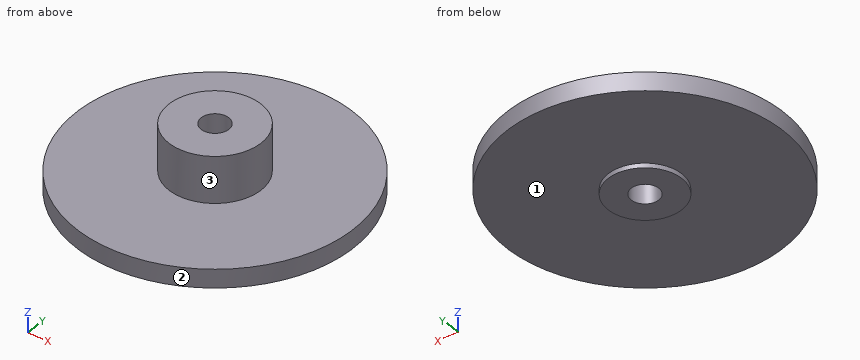
Autodesk Inventor part; units mm, degrees
ref_plane "YZ Plane" through (0, 0, 0) normal (1, 0, 0) x (0, 1, 0)
ref_plane "XZ Plane" through (0, 0, 0) normal (0, 1, 0) x (-1, 0, 0)
ref_plane "XY Plane" through (0, 0, 0) normal (0, 0, 1) x (1, 0, 0)
sketch "スケッチ1" plane through (0, 0, 0) normal (0, 0, 1) x (1, 0, 0)
  circle A0 centre (0, 0) radius 15
  dimension "d0" = 30
extrude "押し出し1" add sketch "スケッチ1" along normal blind 2
sketch "スケッチ2" plane through (0, 0, 2) normal (0, 0, 1) x (1, 0, 0)
  circle A0 centre (0, 0) radius 5
  dimension "d3" = 10
extrude "押し出し2" add sketch "スケッチ2" along normal blind 5
sketch "スケッチ4" plane through (0, 0, 0) normal (0, 0, -1) x (-1, 0, 0)
  circle A0 centre (0, 0) radius 4
  dimension "d9" = 8
extrude "押し出し4" add sketch "スケッチ4" along normal blind 0.5
sketch "スケッチ5" plane through (0, 0, 7) normal (0, 0, 1) x (1, 0, 0)
  circle A0 centre (0, 0) radius 1.5
  dimension "d12" = 3
extrude "押し出し5" cut sketch "スケッチ5" against normal blind 15
properties part number "Gear2_BSS0.5-30A" material "真鍮"
Geometry: final body of the model. Coordinates: model frame, mm. Face numbers are marked on the shaded views. A direction names the side the tool comes from. Give positions to 0.01 mm unless a question says otherwise; leave off trailing zeros. Loops run counter-clockwise (first coordinate to the right, second up) from the corner with the lowest first, then second, coordinate; pieces in that order, holes last. Notation, with made-up numbers: (50.5, 28.25) - (86.5, 28.25) arc R34 cw to (86.5, 63.25) - close; hole circle Ø1 at (-29, 85.25). An arc over 180 degrees is marked (long way). One line per question, with ' | ' between items. Start each with the question number.
(1) Section query A-A on x = 0. Return loops of the section in (y, z).
(2) Ray query, line 1 (Y direction, x = 0, z = 2.5); line 2 (Z direction, x = 5.75, y = 6.5); line 3 (Y direction, x = 0.5, z = 5). Return the intervals inside material, ascending. Write a range as from..to.
(3) Reachability of the marked faces 1, 2 and 3 from +Z, -Z, +X, -X, +Y, -Y: full face, straight path, thin tool, end or side. Return the list, or none.
(4) Section query C-C on z = 4.75. Return loops of the section in (x, y).
(5) Section query D-D on x = -12. Return loops of the section in (y, z).
(6) Contact query for flat-ended pins moving along their axis: pin 1 (3.5 mm diameter, centred on x = 0, y = 0, fed in from +Z); pin 2 (4 mm diameter, centred on x = 6, z = 4.5, fed in from +Y); pin 3 (1 mm diameter, centred on x = 4, z = 6, fed in from +Y); pin 4 (3 mm diameter, centred on y = 0.5, z = 5.5, fed in from -X). Output: stop coordinate, or through.
The answers:
1) outline: (-15, 0) - (-4, 0) - (-4, -0.5) - (-1.5, -0.5) - (-1.5, 7) - (-5, 7) - (-5, 2) - (-15, 2) - close; (1.5, -0.5) - (4, -0.5) - (4, 0) - (15, 0) - (15, 2) - (5, 2) - (5, 7) - (1.5, 7) - close
2) line 1: -5..-1.5, 1.5..5 | line 2: 0..2 | line 3: -4.97..-1.41, 1.41..4.97
3) face 1: -Z | face 2: +Z, -Z | face 3: +Z
4) outline: circle Ø10 at (0, 0); hole circle Ø3 at (0, 0)
5) outline: (-9, 0) - (9, 0) - (9, 2) - (-9, 2) - close
6) pin 1: z = 7 | pin 2: y = 3 | pin 3: y = 3.57 | pin 4: x = -5
